```python
from build123d import *

# Parameters (mm, degrees)
EXTRUDE_1_DEPTH              = 100
HOLE_WIZARD_M2_1_D           = 2.4
HOLE_WIZARD_M2_1_CBORE_D     = 6
HOLE_WIZARD_M2_1_CBORE_DEPTH = 3.5
PATTERN_LINEAR_1_COUNT       = 5
PATTERN_LINEAR_1_PITCH       = 20


with BuildPart() as part:
    # 草图1 → 凸台-拉伸1 (new body)
    with BuildSketch(Plane.XY):
        with BuildLine():
            Line((-4.5, -2.905269119), (-4.5, -6.175269119))
            Line((-4.5, -6.175269119), (-4.174730881, -6.500538239))
            Line((-4.174730881, -6.500538239), (0, -6.500538239))
            Line((0, -6.500538239), (4.174730881, -6.500538239))
            Line((4.174730881, -6.500538239), (4.5, -6.175269119))
            Line((4.5, -6.175269119), (4.5, -2.905269119))
            ThreePointArc((4.5, -2.905269119), (4.188070601, -2.722678698), (3.990111871, -2.420269119))
            Line((3.990111871, -2.420269119), (3.630111871, -2.420269119))
            ThreePointArc((3.630111871, -2.420269119), (3.566472261, -2.39390873), (3.540111871, -2.330269119))
            Line((3.540111871, -2.330269119), (3.540111871, -1.970269119))
            ThreePointArc((3.540111871, -1.970269119), (3.566472261, -1.906629509), (3.630111871, -1.880269119))
            Line((3.630111871, -1.880269119), (3.990111871, -1.880269119))
            ThreePointArc((3.990111871, -1.880269119), (4.188070601, -1.577859541), (4.5, -1.395269119))
            Line((4.5, -1.395269119), (4.5, -0.325269119))
            Line((4.5, -0.325269119), (4.174730881, 0))
            Line((4.174730881, 0), (0, 0))
            Line((0, 0), (-4.174730881, 0))
            Line((-4.174730881, 0), (-4.5, -0.325269119))
            Line((-4.5, -0.325269119), (-4.5, -1.395269119))
            ThreePointArc((-4.5, -1.395269119), (-4.188070601, -1.577859541), (-3.990111871, -1.880269119))
            Line((-3.990111871, -1.880269119), (-3.630111871, -1.880269119))
            ThreePointArc((-3.630111871, -1.880269119), (-3.566472261, -1.906629509), (-3.540111871, -1.970269119))
            Line((-3.540111871, -1.970269119), (-3.540111871, -2.330269119))
            ThreePointArc((-3.540111871, -2.330269119), (-3.566472261, -2.39390873), (-3.630111871, -2.420269119))
            Line((-3.630111871, -2.420269119), (-3.990111871, -2.420269119))
            ThreePointArc((-3.990111871, -2.420269119), (-4.188070601, -2.722678698), (-4.5, -2.905269119))
        make_face()
    extrude(amount=EXTRUDE_1_DEPTH)

    # M2 六角头螺栓的柱形沉头孔1 (through all)
    with Locations(Plane(origin=(0, 0, 0), x_dir=(1, 0, 0), z_dir=(0, 1, 0))):
        with Locations((0, -90)):
            hole_wizard_m2_1 = CounterBoreHole(HOLE_WIZARD_M2_1_D / 2, HOLE_WIZARD_M2_1_CBORE_D / 2, HOLE_WIZARD_M2_1_CBORE_DEPTH)

    # 阵列(线性)1: M2 六角头螺栓的柱形沉头孔1 ×5
    with Locations(*[(0, 0, -i * PATTERN_LINEAR_1_PITCH) for i in range(1, PATTERN_LINEAR_1_COUNT)]):
        add(hole_wizard_m2_1, mode=Mode.SUBTRACT)


solid = part.part
```
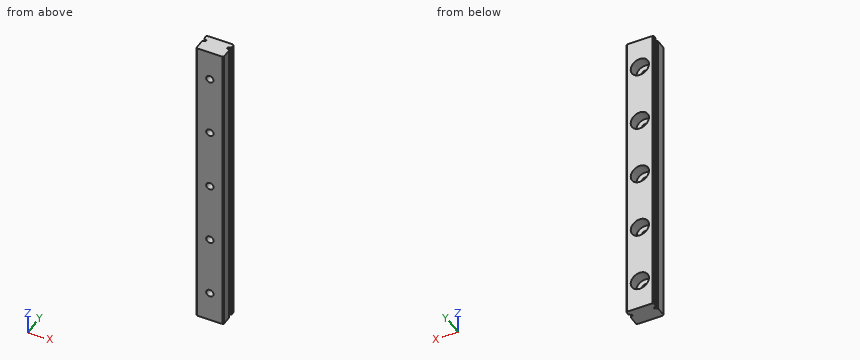
Read the model definition and answer for the solid it produces. Units are mm, in the model's axes. Round coordinates to 2 decimals unless told otherwise and drop trailing zeros. Write each loop counter-clockwise with the first axis right and the second up, starting at its lowest first coordinate (ties: lowest second). Pieces come first, ordered by that corner, then holes. Notation, with made-up numbers: (60.5, 1) -> (66.5, 1) arc R19 ccw to (66.5, 22) -> close; hole circle Ø1 at (79, -27.5). An arc over 180 degrees is marked (long way). Answer in a Markdown table with one row per item. Add a question column.
1) Find section A-A, the plane y = -4.75. Determine the outline of the cut face in (x, z), and give its area (3 significant figures).
2) Consider line 1 (Z direction, x = 0, y = -1.65); line 2 (Z direction, x = 0, y = -5.4); line 3 (X direction, y = -2.2, z = 90). Determine where each line is inside the solid, lowest interval first.
3) Given P1, Ø3, axis at x = -1, z = 70.5, coming from the +Y side, flat-ended and moving along its own axis, determine where the tip first touches the part or whether it passes through.
4) Find section C-C, the plane z = 40.5. Determine the outline of the cut face in (x, y), and give its area (3 significant figures).
5) Find section D-D, the plane x = 0. State how many separate pieces and enclosed holes the cut face has, and give its area (3 significant figures).
Findings below:
| question | item | result |
|---|---|---|
| 1 | outline | (-4.5, 0) -> (4.5, 0) -> (4.5, 100) -> (-4.5, 100) -> close; hole circle Ø2.4 at (0, 10); hole circle Ø2.4 at (0, 30); hole circle Ø2.4 at (0, 50); hole circle Ø2.4 at (0, 70); hole circle Ø2.4 at (0, 90) |
| 1 | area | 877 mm² |
| 2 | line 1 | 0 to 7, 13 to 27, 33 to 47, 53 to 67, 73 to 87, 93 to 100 |
| 2 | line 2 | 0 to 8.8, 11.2 to 28.8, 31.2 to 48.8, 51.2 to 68.8, 71.2 to 88.8, 91.2 to 100 |
| 2 | line 3 | -3.54 to -3, 3 to 3.54 |
| 3 | P1 | y = -3.5 |
| 4 | outline | (-4.5, -6.18) -> (-4.17, -6.5) -> (4.17, -6.5) -> (4.5, -6.18) -> (4.5, -2.91) arc R0.79 cw to (3.99, -2.42) -> (3.63, -2.42) arc R0.09 cw to (3.54, -2.33) -> (3.54, -1.97) arc R0.09 cw to (3.63, -1.88) -> (3.99, -1.88) arc R0.79 cw to (4.5, -1.4) -> (4.5, -0.33) -> (4.17, 0) -> (-4.17, 0) -> (-4.5, -0.33) -> (-4.5, -1.4) arc R0.79 cw to (-3.99, -1.88) -> (-3.63, -1.88) arc R0.09 cw to (-3.54, -1.97) -> (-3.54, -2.33) arc R0.09 cw to (-3.63, -2.42) -> (-3.99, -2.42) arc R0.79 cw to (-4.5, -2.91) -> close |
| 4 | area | 56.6 mm² |
| 5 | separate pieces | 6 |
| 5 | enclosed holes | 0 |
| 5 | area | 509 mm² |
